Check sheet for the modelled part. Datum: model origin and axes. Units: mm. Coordinates: 2 decimals unless noted, no trailing zeros. Order: outer loops, then holes, each group sorted by start corner. A loop starts at its lowest first (then second) coordinate and runs counter-clockwise, first axis right, second up.
Autodesk Inventor part; units mm, degrees
ref_plane "YZ Plane" through (0, 0, 0) normal (1, 0, 0) x (0, 1, 0)
ref_plane "XZ Plane" through (0, 0, 0) normal (0, 1, 0) x (-1, 0, 0)
ref_plane "XY Plane" through (0, 0, 0) normal (0, 0, 1) x (1, 0, 0)
sketch "Sketch1" plane through (0, 0, 0) normal (0, 1, 0) x (-1, 0, 0)
  line L0 (63.5, -101.6) -> (-63.5, -101.6)
  line L1 (-63.5, -101.6) -> (-63.5, 101.6)
  line L2 (-63.5, 101.6) -> (63.5, 101.6)
  line L3 (63.5, 101.6) -> (63.5, -101.6)
  line L4 (63.5, -101.6) -> (-63.5, 101.6) construction
  line L5 (-63.5, -101.6) -> (63.5, 101.6) construction
  circle A0 centre (36.3684, -65.2364) radius 11.6586
  line L6 (57.15, 95.25) -> (-57.15, 95.25)
  line L7 (-57.15, 95.25) -> (-57.15, -95.25)
  line L8 (-57.15, -95.25) -> (57.15, -95.25)
  line L9 (57.15, -95.25) -> (57.15, 95.25)
  line L10 (57.15, 95.25) -> (-57.15, -95.25) construction
  line L11 (-57.15, 95.25) -> (57.15, -95.25) construction
  point P0 (0, 0)
  dimension "d0" = 127
  dimension "d1" = 203.2
  dimension "d4" = 23.3172
  dimension "d7" = 114.3
  dimension "d8" = 190.5
extrude "Extrusion2" add sketch "Sketch1" along normal blind 6.35 contours L0 L1 L2 L3 | L9 L8 L7 L6
hole "Hole1" at (57.15, 0, -95.25) at (-57.15, 0, -95.25) at (-57.15, 0, 95.25) at (57.15, 0, 95.25) direction (0, 1, 0) diameter 6.35 end through all
properties part number "eboardpartisland"
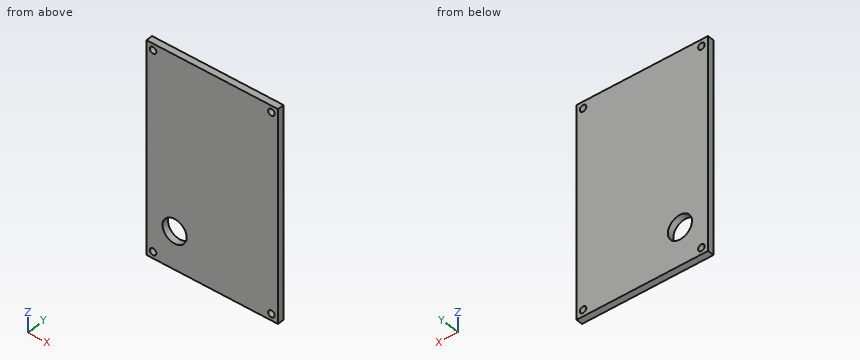
(1) Cross-section at C-C (y = 2.25). Enter the section's corners in (x, z) (3 decimals), and give its area (3 significant figures).
Filled in:
outline: (-63.5, -101.6) - (63.5, -101.6) - (63.5, 101.6) - (-63.5, 101.6) - close; hole circle Ø6.35 at (-57.15, -95.25); hole circle Ø6.35 at (-57.15, 95.25); hole circle Ø23.317 at (-36.368, -65.236); hole circle Ø6.35 at (57.15, -95.25); hole circle Ø6.35 at (57.15, 95.25)
area: 25,300 mm2
(2) Cross-section at D-D (x = -42). Enter the section's corners in (y, z).
Filled in:
outline: (0, -101.6) - (6.35, -101.6) - (6.35, -75.44) - (0, -75.44) - close; (0, -55.03) - (6.35, -55.03) - (6.35, 101.6) - (0, 101.6) - close
(3) Cross-section at A-A (x = 57.15). Enter the section's corners in (y, z) (3 decimals).
Filled in:
outline: (0, -101.6) - (6.35, -101.6) - (6.35, -98.425) - (0, -98.425) - close; (0, -92.075) - (6.35, -92.075) - (6.35, 92.075) - (0, 92.075) - close; (0, 98.425) - (6.35, 98.425) - (6.35, 101.6) - (0, 101.6) - close
(4) Cross-section at B-B (z = 95.25). Enter the section's corners in (x, y) (3 decimals), and give its area (3 significant figures).
Filled in:
outline: (-63.5, 0) - (-60.325, 0) - (-60.325, 6.35) - (-63.5, 6.35) - close; (-53.975, 0) - (53.975, 0) - (53.975, 6.35) - (-53.975, 6.35) - close; (60.325, 0) - (63.5, 0) - (63.5, 6.35) - (60.325, 6.35) - close
area: 726 mm2
(5) Go/stop test with a flat-tipped pin: P1, Ø4, axis at x = 57.15, z = -95.25, coming from the -Y side. Record where the tip stops, or that it passes through.
Filled in:
P1: passes through
(6) Thickness scan on probe 1 along Z at (x, y) = (57.15, 2) (3 decimals); probe 2 along X at (y, z) = (2.5, -95.25) (3 decimals); probe 3 along Z at (x, y) = (-29, 4). Record the ranges inside material, lowest first.
Filled in:
probe 1: z = -101.6 to -98.425, -92.075 to 92.075, 98.425 to 101.6
probe 2: x = -63.5 to -60.325, -53.975 to 53.975, 60.325 to 63.5
probe 3: z = -101.6 to -74.27, -56.2 to 101.6
